Geometry: see drawing. Coordinates: mm, zero at the bounding-box minimum. A direction names the side the tool comes from. Give positions to 0.01 mm unless a question says otherwise; leave off trailing zeros. Order: outer loops, then holes, each group sorted by start corner. A loop starts at its lowest first (then second) coordinate and runs counter-clockwise, first axis right, second up. Notation, with made-up numbers: (21.5, -14) - (52.5, -14) arc R13 ccw to (52.5, 10) - close; hole circle Ø11 at (16, 74). An arc over 180 degrees is marked (long way). Write each question's results on one line, items separated by ' | '. Start each with the question number.
Item 1: Section B-B on z = 12.5. Output: boundary loops of the cut face in (x, y), and give its area (3 significant figures).
Item 2: Line query: line 1 along Y through (x, z) = (4, 16.25); line 2 along X through (y, z) = (26, 12.25); line 3 along X through (y, z) = (57, 5). Output: solid intervals per line, ascending.
Item 3: Contact query for flat-ended pins moving along their axis: pin 1 Ø1.3 at (x, y) = (12.5, 80.5) entering from -Z; pin 2 Ø1 at (x, z) = (5, 2.5) entering from +Y; pin 3 Ø6 at (y, z) = (64.5, 5.5) entering from -X. Output: stop coordinate, or through.
Item 4: Set-up query: the marked faces 1 and 2. Return all of +Z, -Z, +X, -X, +Y, -Y with unobstructed straight access to the full face (end or side cutting, diameter ignored); none if empty.
Item 5: Section C-C on y = 63. Output: boundary loops of the cut face in (x, z).
Item 6: Section D-D on y = 21.5. Output: boundary loops of the cut face in (x, z).
Item 7: Section A-A on x = 12.5. Output: boundary loops of the cut face in (y, z), and give its area (3 significant figures).
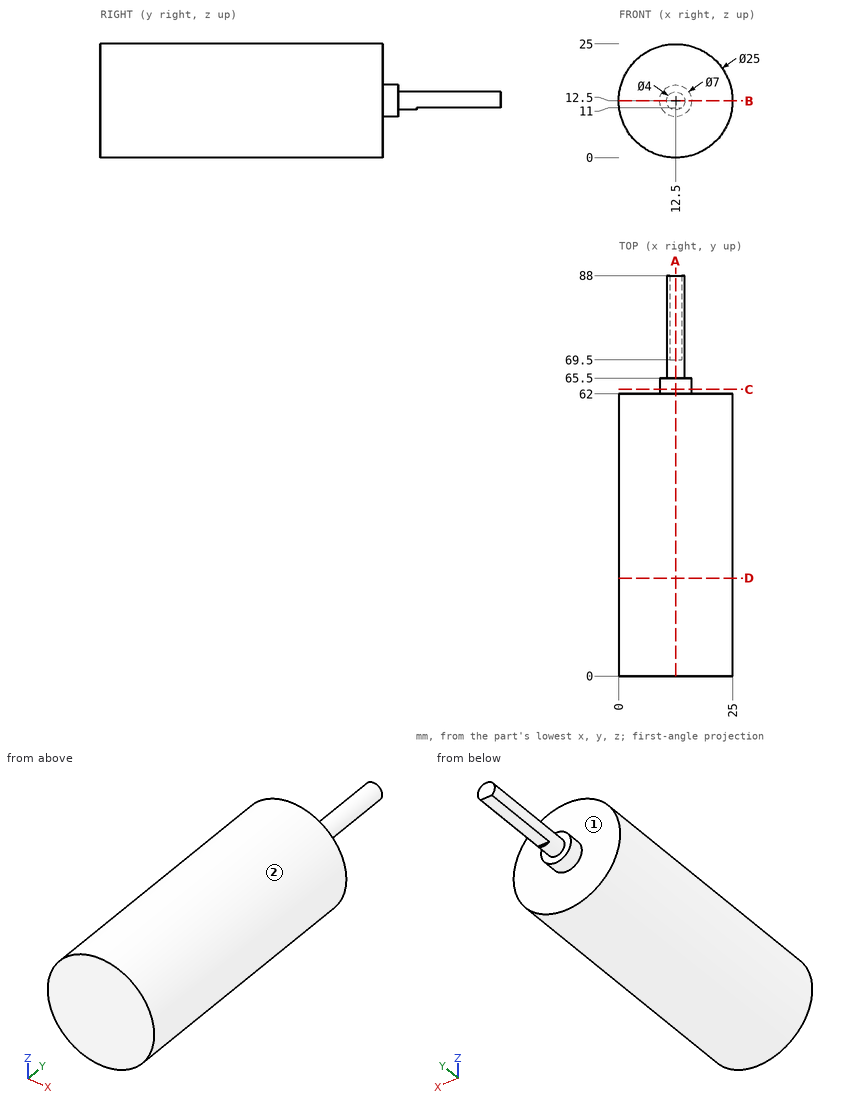
Evaluation:
1) outline: (0, 0) - (25, 0) - (25, 62) - (16, 62) - (16, 65.5) - (14.5, 65.5) - (14.5, 88) - (10.5, 88) - (10.5, 65.5) - (9, 65.5) - (9, 62) - (0, 62) - close | area: 1,660 mm^2
2) line 1: y = 0 to 62 | line 2: x = 0 to 25 | line 3: x = 2.5 to 22.5
3) pin 1: stops at z = 11 | pin 2: stops at y = 62 | pin 3: stops at x = 1.2
4) face 1: +Y | face 2: +Y, -Y
5) outline: circle Ø7 at (12.5, 12.5)
6) outline: circle Ø25 at (12.5, 12.5)
7) outline: (0, 0) - (62, 0) - (62, 9) - (65.5, 9) - (65.5, 10.5) - (69.5, 10.5) - (69.5, 11) - (88, 11) - (88, 14.5) - (65.5, 14.5) - (65.5, 16) - (62, 16) - (62, 25) - (0, 25) - close | area: 1,660 mm^2
